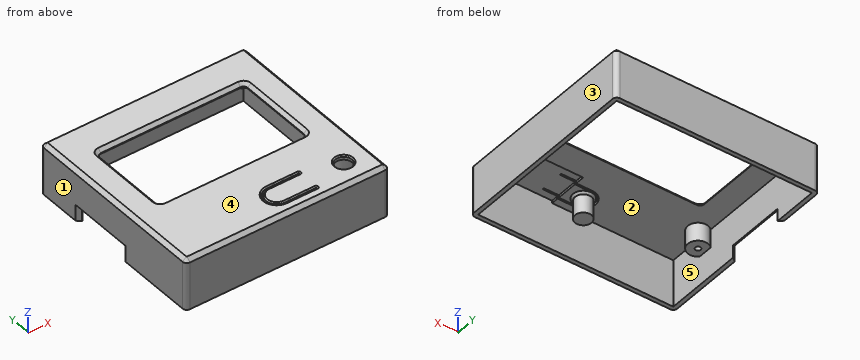
from build123d import *

# Parameters (mm, degrees)
SKETCH001018_W   = 99
SKETCH001018_H   = 93
PAD013_DEPTH     = 2
SKETCH001019_R   = 4
POCKET004_DEPTH  = 2.001
SKETCH001020_W   = 99
SKETCH001020_H   = 93
SKETCH001020_W_2 = 95
SKETCH001020_H_2 = 89
PAD014_DEPTH     = 23
PAD015_DEPTH     = 8.9
SKETCH001022_R   = 1.3
POCKET005_DEPTH  = 8.9
FILLET004_R      = 2
CHAMFER001_SIZE  = 1.8
CHAMFER002_SIZE  = 1.6
SKETCH001023_R   = 4
PAD016_DEPTH     = 10
CHAMFER003_SIZE  = 1
SKETCH001024_W   = 20
SKETCH001024_H   = 20
POCKET006_DEPTH  = 1.2
SKETCH001025_W   = 4
SKETCH001025_H   = 28.5
POCKET007_DEPTH  = 6.1
CHAMFER004_SIZE  = 1.8
CHAMFER005_SIZE  = 0.6
CHAMFER006_SIZE  = 0.6


with BuildPart() as part:
    # Sketch001018 → Pad013 (new body)
    with BuildSketch(Plane.XY.offset(15.2)):
        Rectangle(SKETCH001018_W, SKETCH001018_H)
    extrude(amount=PAD013_DEPTH)

    # Sketch001019 → Pocket004 (cut, through all)
    with BuildSketch(Plane.XY.offset(17.2)):
        with Locations((36.5, -34.5)):
            Circle(SKETCH001019_R)
        with BuildLine():
            Line((-34, 28.5), (34, 28.5))
            ThreePointArc((36, 26.5), (35.414214, 27.914214), (34, 28.5))
            Line((36, 26.5), (36, -9.5))
            ThreePointArc((34, -11.5), (35.414214, -10.914214), (36, -9.5))
            Line((34, -11.5), (-34, -11.5))
            ThreePointArc((-36, -9.5), (-35.414214, -10.914214), (-34, -11.5))
            Line((-36, -9.5), (-36, 26.5))
            ThreePointArc((-34, 28.5), (-35.414214, 27.914214), (-36, 26.5))
        make_face()
        with BuildLine():
            ThreePointArc((3.5, -29.8), (-1.7, -35), (3.5, -40.2))
            Line((3.5, -40.2), (18.5, -40.2))
            ThreePointArc((18.5, -41), (18.9, -40.6), (18.5, -40.2))
            Line((3.500001, -41), (18.5, -41))
            ThreePointArc((3.5, -29), (-2.5, -35), (3.500001, -41))
            Line((3.5, -29), (18.5, -29))
            ThreePointArc((18.499999, -29.8), (18.9, -29.4), (18.5, -29))
            Line((3.5, -29.8), (18.499999, -29.8))
        make_face()
    extrude(amount=-POCKET004_DEPTH, mode=Mode.SUBTRACT)

    # Sketch001020 → Pad014 (new body)
    with BuildSketch(Plane(origin=(0, 0, 15.2), x_dir=(1, 0, 0), z_dir=(0, 0, -1))):
        Rectangle(SKETCH001020_W, SKETCH001020_H)
        Rectangle(SKETCH001020_W_2, SKETCH001020_H_2, mode=Mode.SUBTRACT)
    extrude(amount=PAD014_DEPTH)

    # Sketch001021 → Pad015 (new body)
    with BuildSketch(Plane(origin=(0, 0, 15.2), x_dir=(1, 0, 0), z_dir=(0, 0, -1))):
        with BuildLine():
            ThreePointArc((-40.429286, -44.5), (-40.464466, -37.464466), (-47.5, -37.429286))
            Line((-47.5, -37.429286), (-47.5, -44.5))
            Line((-47.5, -44.5), (-40.429286, -44.5))
        make_face()
        with BuildLine():
            ThreePointArc((-47.5, 20.429286), (-39, 24), (-47.5, 27.570714))
            Line((-47.5, 27.570714), (-47.5, 20.429286))
        make_face()
        with BuildLine():
            ThreePointArc((47.5, 27.570714), (39, 24), (47.5, 20.429286))
            Line((47.5, 27.570714), (47.5, 20.429286))
        make_face()
        with BuildLine():
            ThreePointArc((47.5, -37.429286), (40.464466, -37.464466), (40.429286, -44.5))
            Line((47.5, -44.5), (40.429286, -44.5))
            Line((47.5, -37.429286), (47.5, -44.5))
        make_face()
    extrude(amount=PAD015_DEPTH)

    # Sketch001022 → Pocket005 (cut)
    with BuildSketch(Plane(origin=(0, 0, 6.3), x_dir=(1, 0, 0), z_dir=(0, 0, -1))):
        with Locations((-44, 24)):
            Circle(SKETCH001022_R)
        with Locations((44, 24)):
            Circle(SKETCH001022_R)
        with Locations((-44, -41)):
            Circle(SKETCH001022_R)
        with Locations((44, -41)):
            Circle(SKETCH001022_R)
    extrude(amount=-POCKET005_DEPTH, mode=Mode.SUBTRACT)

    # Fillet004
    fillet004_edges = [part.edges().sort_by_distance(p)[0] for p in [
        (-49.5, -46.5, 3.7),
        (-49.5, -46.5, 16.2),
        (-49.5, 46.5, 16.2),
        (-49.5, 46.5, 3.7),
        (49.5, 46.5, 16.2),
        (49.5, 46.5, 3.7),
        (49.5, -46.5, 16.2),
        (49.5, -46.5, 3.7),
    ]]
    fillet(fillet004_edges, radius=FILLET004_R)

    # Chamfer001
    chamfer001_edges = [part.edges().sort_by_distance(p)[0] for p in [
        (0, -46.5, 17.2),
        (-48.914214, -45.914214, 17.2),
        (-49.5, 0, 17.2),
        (48.914214, -45.914214, 17.2),
        (49.5, 0, 17.2),
        (48.914214, 45.914214, 17.2),
        (0, 46.5, 17.2),
        (-48.914214, 45.914214, 17.2),
    ]]
    chamfer(chamfer001_edges, length=CHAMFER001_SIZE)

    # Chamfer002
    chamfer002_edges = [part.edges().sort_by_distance(p)[0] for p in [
        (0, 28.5, 17.2),
        (35.414214, 27.914214, 17.2),
        (36, 8.5, 17.2),
        (35.414214, -10.914214, 17.2),
        (-35.414214, 27.914214, 17.2),
        (-36, 8.5, 17.2),
        (-35.414214, -10.914214, 17.2),
        (0, -11.5, 17.2),
    ]]
    chamfer(chamfer002_edges, length=CHAMFER002_SIZE)

    # Sketch001023 → Pad016 (new body)
    with BuildSketch(Plane(origin=(0, 0, 15.2), x_dir=(1, 0, 0), z_dir=(0, 0, -1))):
        with Locations((3.5, 35)):
            Circle(SKETCH001023_R)
    extrude(amount=PAD016_DEPTH)

    # Chamfer003
    chamfer003_edges = [part.edges().sort_by_distance(p)[0] for p in [
        (-0.5, -35, 15.2),
    ]]
    chamfer(chamfer003_edges, length=CHAMFER003_SIZE)

    # Sketch001024 → Pocket006 (cut)
    with BuildSketch(Plane(origin=(0, 0, 15.2), x_dir=(1, 0, 0), z_dir=(0, 0, -1))):
        with Locations((21.5, 34.5)):
            Rectangle(SKETCH001024_W, SKETCH001024_H)
    extrude(amount=-POCKET006_DEPTH, mode=Mode.SUBTRACT)

    # Sketch001025 → Pocket007 (cut)
    with BuildSketch(Plane(origin=(0, 0, -7.8), x_dir=(1, 0, 0), z_dir=(0, 0, -1))):
        with Locations((-48.5, -8.25)):
            Rectangle(SKETCH001025_W, SKETCH001025_H)
    extrude(amount=-POCKET007_DEPTH, mode=Mode.SUBTRACT)

    # Chamfer004
    chamfer004_edges = [part.edges().sort_by_distance(p)[0] for p in [
        (-49.5, -6, -4.75),
        (-49.5, 8.25, -1.7),
        (-49.5, 22.5, -4.75),
    ]]
    chamfer(chamfer004_edges, length=CHAMFER004_SIZE)

    # Chamfer005
    chamfer005_edges = [part.edges().sort_by_distance(p)[0] for p in [
        (11, -29.8, 17.2),
        (18.9, -29.4, 17.2),
        (11, -29, 17.2),
        (-2.5, -35, 17.2),
        (-1.7, -35, 17.2),
        (11, -40.2, 17.2),
        (11, -41, 17.2),
        (18.9, -40.6, 17.2),
    ]]
    chamfer(chamfer005_edges, length=CHAMFER005_SIZE)

    # Chamfer006
    chamfer006_edges = [part.edges().sort_by_distance(p)[0] for p in [
        (32.5, -34.5, 17.2),
    ]]
    chamfer(chamfer006_edges, length=CHAMFER006_SIZE)


solid = part.part
Can you work these out from the model? Positions are in its coordinate system, mm. Face numbers are marked on the shaded views. A direction names the side the tool comes from. Give positions to 0.01 mm unless a question says otherwise; leave off trailing zeros. Write each loop counter-clockwise with the first axis right and the second up, starting at its lowest first coordinate (ties: lowest second). Pieces come first, ordered by that corner, then holes. Notation, with made-up numbers: (66.25, -14.5) -> (92.25, -14.5) arc R25 cw to (92.25, 22.5) -> close; hole circle Ø11 at (57, 31.5). An arc over 180 degrees is marked (long way). Answer as a JSON object with one key per item and string values. Group by question number.
Item 1: I'm going to push flat-ended pins straight in: P1, Ø8.5, axis at x = 5.5, y = -32.5, coming from the -Z side; P2, Ø0.6, axis at y = -43, z = 16, coming from the +X side; P3, Ø2.5, axis at x = 43.5, y = -23.5, coming from the -Z side. Where does each tip first touch, or does it pass through?
Item 2: Suppose I cut it at A-A (y = 6). Please give me the cut outline in (x, z), plus the area to 3 significant figures.
Item 3: Suppose I cut it at C-C (x = -24). Please give me the cut outline in (y, z).
Item 4: Suppose I cut it at B-B (z = 3.75). Please give me the cut outline in (x, y).
Item 5: We'd pull the mould along X, two halves only. Please class the marked faces 1, 2 and 3: +X half, -X half, draft (parallel to the pull), parting line (faces both ways), or undercut.
Item 6: For the marked faces 4 and 5, which set-ups out of +Z, -Z, +X, -X, +Y, -Y let a thin tool reach every point of the face, with its end or its side?
Item 7: Suppose I cut it at D-D (z = 11.25). Please give me the cut outline in (x, y), plus the area to 3 significant figures.
Item 8: Please list where these lines run through material, in increasing order: line 1 (X direction, y = -24, z = 12.5); line 2 (Y direction, x = -44, z = 9.5); line 3 (X direction, y = 35, z = 1.75). Write a range as [from, to].
Findings:
{
 "1": {"P1": "stops at z = 5.2", "P2": "stops at x = 49.2", "P3": "stops at z = 6.3"},
 "2": {"outline": "(-49.5, 0.1) -> (-47.7, -1.7) -> (-47.5, -1.7) -> (-47.5, 15.2) -> (-36, 15.2) -> (-36, 15.6) -> (-37.6, 17.2) -> (-47.7, 17.2) -> (-49.5, 15.4) -> close; (36, 15.2) -> (47.5, 15.2) -> (47.5, -7.8) -> (49.5, -7.8) -> (49.5, 15.4) -> (47.7, 17.2) -> (37.6, 17.2) -> (36, 15.6) -> close", "area": "126 mm²"},
 "3": {"outline": "(-46.5, -7.8) -> (-44.5, -7.8) -> (-44.5, 15.2) -> (-11.5, 15.2) -> (-11.5, 15.6) -> (-13.1, 17.2) -> (-44.7, 17.2) -> (-46.5, 15.4) -> close; (28.5, 15.2) -> (44.5, 15.2) -> (44.5, -7.8) -> (46.5, -7.8) -> (46.5, 15.4) -> (44.7, 17.2) -> (30.1, 17.2) -> (28.5, 15.6) -> close"},
 "4": {"outline": "(-49.5, -44.5) arc R2 ccw to (-47.5, -46.5) -> (47.5, -46.5) arc R2 ccw to (49.5, -44.5) -> (49.5, 44.5) arc R2 ccw to (47.5, 46.5) -> (-47.5, 46.5) arc R2 ccw to (-49.5, 44.5) -> close; hole (-47.5, -44.5) -> (47.5, -44.5) -> (47.5, 44.5) -> (-47.5, 44.5) -> close"},
 "5": {"face 1": "-X half", "face 2": "undercut", "face 3": "+X half"},
 "6": {"face 4": "+Z, +X, -X, +Y, -Y", "face 5": "-Z"},
 "7": {"outline": "(-49.5, -44.5) arc R2 ccw to (-47.5, -46.5) -> (47.5, -46.5) arc R2 ccw to (49.5, -44.5) -> (49.5, 44.5) arc R2 ccw to (47.5, 46.5) -> (-47.5, 46.5) arc R2 ccw to (-49.5, 44.5) -> close; circle Ø8 at (3.5, -35); hole (-47.5, -44.5) -> (47.5, -44.5) -> (47.5, -27.57) arc R5 cw (long way) to (47.5, -20.43) -> (47.5, 37.43) arc R5 cw to (40.43, 44.5) -> (-40.43, 44.5) arc R5 cw to (-47.5, 37.43) -> (-47.5, -20.43) arc R5 cw (long way) to (-47.5, -27.57) -> close; hole circle Ø2.6 at (-44, -24); hole circle Ø2.6 at (-44, 41); hole circle Ø2.6 at (44, -24); hole circle Ø2.6 at (44, 41)", "area": "1,050 mm²"},
 "8": {"line 1": "x = [-49.5, -45.3], [-42.7, -39], [39, 42.7], [45.3, 49.5]", "line 2": "y = [-46.5, -44.5], [-29, -25.3], [-22.7, -19], [36, 39.7], [42.3, 46.5]", "line 3": "x = [-49.5, -47.5], [47.5, 49.5]"}
}
